Verification items for the finished model (mm, model axes). Face numbers are marked on the shaded views. A direction names the side the tool comes from. Round coordinates to 2 decimals unless told otherwise and drop trailing zeros. Order: outer loops, then holes, each group sorted by start corner. A loop starts at its lowest first (then second) coordinate and runs counter-clockwise, first axis right, second up. Notation, with made-up numbers: M 62,23.5 L 86,23.5 A15 cw 86,40.5 Z; hole C 38.5,28.25 d5. An arc over 180 degrees is marked long. Return JSON: item names as keys, results as strings. Group by question number.
from build123d import *

# Parameters (mm, degrees)
SKETCH1_R           = 20
BOSS_EXTRUDE1_DEPTH = 40
SKETCH2_R           = 7.5
CUT_EXTRUDE1_DEPTH  = 10
SKETCH3_W           = 33.40458463
SKETCH3_H           = 9.314739944
CUT_EXTRUDE2_DEPTH  = 10


with BuildPart() as part:
    # Sketch1 → Boss-Extrude1 (new body)
    with BuildSketch(Plane(origin=(0, 0, 0), x_dir=(1, 0, 0), z_dir=(0, 1, 0))):
        Circle(SKETCH1_R)
    extrude(amount=BOSS_EXTRUDE1_DEPTH)

    # Sketch2 → Cut-Extrude1 (cut)
    with BuildSketch(Plane(origin=(0, 40, 0), x_dir=(1, 0, 0), z_dir=(0, 1, 0))):
        Circle(SKETCH2_R)
    extrude(amount=-CUT_EXTRUDE1_DEPTH, mode=Mode.SUBTRACT)

    # Sketch3 → Cut-Extrude2 (cut)
    with BuildSketch(Plane.XY.offset(-20)):
        with Locations((0, 20.883294305)):
            Rectangle(SKETCH3_W, SKETCH3_H)
    extrude(amount=CUT_EXTRUDE2_DEPTH, mode=Mode.SUBTRACT)


solid = part.part
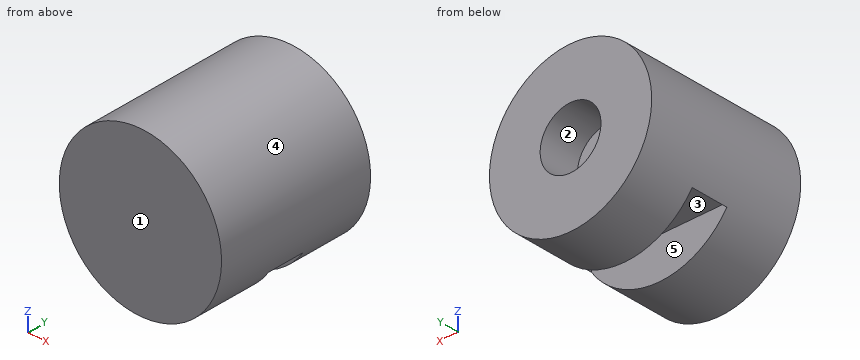
1. Thickness scan on line 1 along Z through (x, y) = (0, 32); line 2 along Y through (x, z) = (4, -15); line 3 along X through (y, z) = (36, -5.5). Record the ranges inside material, lowest first. Write a range as from..to.
2. Go/stop test with flat-tipped pins: pin 1 (5 mm diameter, centred on y = 12.5, z = -6, fed in from +X); pin 2 (8 mm diameter, centred on y = 32, z = 4.5, fed in from -X); pin 3 (6 mm diameter, centred on x = -11.5, y = 20, fed in from +Z). Record where each tip stops, or that it passes through.
3. Cross-section at C-C (y = 9). Enter the section's corners in (x, z).
4. Cross-section at B-B (x = 0). Enter the section's corners in (y, z), plus the area to 3 significant figures.
5. Cross-section at A-A (z = 0). Enter the section's corners in (x, y), plus the area to 3 significant figures.
6. Draft check along Z on the marked faces 1, 2 and 3. Enter one of: +Z half, -Z half, draft (parallel to the pull), parting line (faces both ways), or undercut.
7. Cross-section at D-D (x = -4.5). Enter the section's corners in (y, z), plus the area to 3 significant figures.
8. Access from +Z, -Z, +X, -X, +Y, -Y to the whole of each face (thin tool, end or side, straight path). Record for the marked faces 4 and 5.
Computed:
{
 "1": {"line 1": "z = -20..-7.5, 7.5..20", "line 2": "y = 0..16.23, 25.54..40", "line 3": "x = -19.23..-5.1, 5.1..19.23"},
 "2": {"pin 1": "stops at x = 19.69", "pin 2": "stops at x = -19.99", "pin 3": "stops at z = 18.1"},
 "3": {"outline": "C 0,0 d40"},
 "4": {"outline": "M 0,-20 L 16.23,-20 L 16.23,-10 L 25.54,-10 L 25.54,-20 L 40,-20 L 40,-7.5 L 30,-7.5 L 30,7.5 L 40,7.5 L 40,20 L 0,20 Z", "area": "1,360 mm²"},
 "5": {"outline": "M -20,0 L 20,0 L 20,40 L 7.5,40 L 7.5,30 L -7.5,30 L -7.5,40 L -20,40 Z", "area": "1,450 mm²"},
 "6": {"face 1": "draft", "face 2": "undercut", "face 3": "-Z half"},
 "7": {"outline": "M 0,-19.49 L 16.23,-19.49 L 16.23,-10 L 25.54,-10 L 25.54,-19.49 L 40,-19.49 L 40,-6 L 30,-6 L 30,6 L 40,6 L 40,19.49 L 0,19.49 Z", "area": "1,350 mm²"},
 "8": {"face 4": "+Y, -Y", "face 5": "-Z"}
}
